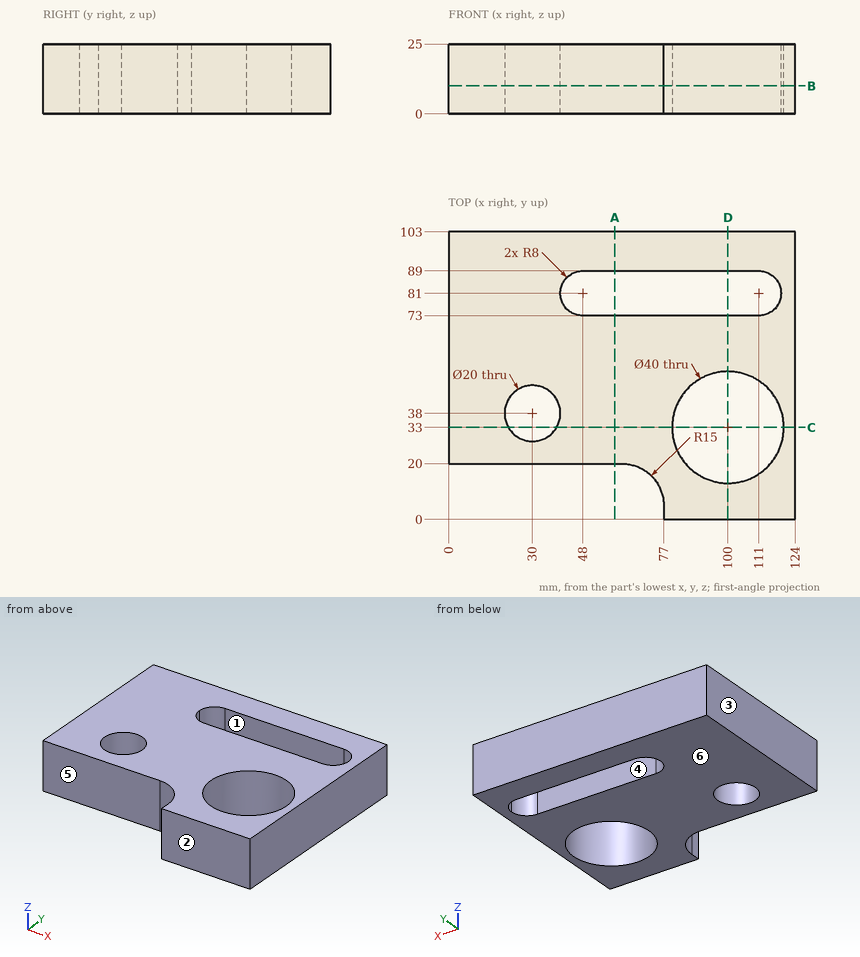
For this review, use the dimensioned drawing (mm, ordinates from the lowest corner) and the shaded views. A direction names the side the tool comes from. Give positions to 0.01 mm unless a question says otherwise; leave off trailing zeros. Loops run counter-clockwise (first coordinate to the right, second up) from the corner with the lowest first, then second, coordinate; pieces in that order, holes last. Notation, with made-up numbers: (84, 20) -> (115, 20) arc R35 cw to (115, 58) -> close; hole circle Ø4 at (16.5, 2). An arc over 180 degrees is marked (long way). One line per question, with ' | ' between items. Start each with the question number.
(1) We need section A-A (x = 59.5). State the section outline as (y, z) points, and give its area (4 significant figures).
(2) Insertion check: P1, Ø3, axis at x = 20, z = 7, coming from the -Y side; P2, Ø1.5, axis at y = 3, z = 8, coming from the -X side. Each pin has a flat end and moves straight along its axis. Give the tip position at first contact, or say it passes through.
(3) We need section B-B (z = 10). State the section outline as (x, y) points.
(4) We need section C-C (y = 33). State the section outline as (x, z) points.
(5) For the marked faces 4, 5 and 6, list the 3-axis set-ups (+Z, -Z, +X, -X, +Y, -Y) from which the entire face can be reached by the end or side of a thin tool; tool diameter is ignored.
(6) For line 1 (Y direction, x = 100, z = 17.5); line 2 (Y direction, x = 30, z = 9.75); line 3 (X direction, y = 44, z = 8.75), list the stretches that pass through material, from the lowest coordinate up.
(7) We need section D-D (x = 100). State the section outline as (y, z) points.
(8) Draft analysis for pull direction Y (two halves, no side actions). For the marked faces 1, 2 and 3, state which applies: +Y half, -Y half, draft (parallel to the pull), parting line (faces both ways), or undercut.
The answers:
1) outline: (20, 0) -> (73, 0) -> (73, 25) -> (20, 25) -> close; (89, 0) -> (103, 0) -> (103, 25) -> (89, 25) -> close | area: 1,675 mm^2
2) P1: stops at y = 20 | P2: stops at x = 77
3) outline: (0, 20) -> (62, 20) arc R15 cw to (77, 5) -> (77, 0) -> (124, 0) -> (124, 103) -> (0, 103) -> close; hole circle Ø20 at (30, 38); hole (40, 81) arc R8 ccw to (48, 73) -> (111, 73) arc R8 ccw to (119, 81) arc R8 ccw to (111, 89) -> (48, 89) arc R8 ccw to start; hole circle Ø40 at (100, 33)
4) outline: (0, 0) -> (21.34, 0) -> (21.34, 25) -> (0, 25) -> close; (38.66, 0) -> (80, 0) -> (80, 25) -> (38.66, 25) -> close; (120, 0) -> (124, 0) -> (124, 25) -> (120, 25) -> close
5) face 4: +Z, -Z | face 5: +Z, -Z, -X, -Y | face 6: -Z, +X, -X, +Y, -Y
6) line 1: y = 0 to 13, 53 to 73, 89 to 103 | line 2: y = 20 to 28, 48 to 103 | line 3: x = 0 to 22, 38 to 83.3, 116.7 to 124
7) outline: (0, 0) -> (13, 0) -> (13, 25) -> (0, 25) -> close; (53, 0) -> (73, 0) -> (73, 25) -> (53, 25) -> close; (89, 0) -> (103, 0) -> (103, 25) -> (89, 25) -> close
8) face 1: undercut | face 2: -Y half | face 3: draft
